Autodesk Fusion 360 part; units mm, degrees
sketch "Esboço3" plane through (0, 0, 0) normal (0, 0, 1) x (1, 0, 0)
box "Primitiva de caixa2" add length 60 width 30 height 5 placed x (0, 1, 0) y (-1, 0, 0) z (0, 0, 1) at (30, 0, 0)
cylinder "Cilindro primitivo2" cut diameter 10 height -35 placed x (1, 0, 0) y (0, 1, 0) z (0, 0, 1) at (15, 15, 5)
cylinder "Cilindro primitivo3" cut diameter 10 height -8 placed x (1, 0, 0) y (0, 1, 0) z (0, 0, 1) at (15, 45, 5)
Work out the finished part from the listing and answer in its coordinate system (mm). Round coordinates to 2 decimals unless told otherwise and drop trailing zeros. Order: outer loops, then holes, each group sorted by start corner. A loop starts at its lowest first (then second) coordinate and runs counter-clockwise, first axis right, second up.
Q1. A cutting plane is placed at D-D, the plane y = 12. Determine the outline of the cut face in (x, z).
Solution:
outline: (0, 0) - (11, 0) - (11, 5) - (0, 5) - close; (19, 0) - (30, 0) - (30, 5) - (19, 5) - close
Q2. A cutting plane is placed at C-C, the plane x = 15. Determine the outline of the cut face in (y, z).
Solution:
outline: (0, 0) - (10, 0) - (10, 5) - (0, 5) - close; (20, 0) - (40, 0) - (40, 5) - (20, 5) - close; (50, 0) - (60, 0) - (60, 5) - (50, 5) - close
Q3. Find the intervals of material crossed by line 1 along Y through (x, z) = (15, 1.6); line 2 along Y through (x, z) = (13.5, 2.7); line 3 along X through (y, z) = (41, 2.05), in increasing order.
Solution:
line 1: y = 0 to 10, 20 to 40, 50 to 60
line 2: y = 0 to 10.23, 19.77 to 40.23, 49.77 to 60
line 3: x = 0 to 12, 18 to 30
Q4. The mould has two halves that part along Y. Classify faces 1 (the flat face through (15, 60, 2)), 2 (the flat face through (30, 30, 2)), 3 (the cylindrical face through (17.307, 10.564, 2.535)): pulls with the +Y half, pulls with the -Y half, needs draft (parallel to the pull), parting line crosses it, or undercut.
Solution:
face 1: pulls with the +Y half
face 2: needs draft
face 3: undercut
Q5. A cutting plane is placed at A-A, the plane y = 41. Determine the outline of the cut face in (x, z).
Solution:
outline: (0, 0) - (12, 0) - (12, 5) - (0, 5) - close; (18, 0) - (30, 0) - (30, 5) - (18, 5) - close
Q6. Given pin 1 Ø1.5 at (x, y) = (12, 44.5) entering from -Z, flat-ended and moving along its own axis, determine where the tip first touches the part or whether it passes through.
Solution:
pin 1: passes through
Q7. A cutting plane is placed at B-B, the plane z = 1.6. Determine the outline of the cut face in (x, y), then the cut area to 3 significant figures.
Solution:
outline: (0, 0) - (30, 0) - (30, 60) - (0, 60) - close; hole circle Ø10 at (15, 15); hole circle Ø10 at (15, 45)
area: 1,640 mm2
